```python
from build123d import *

# Parameters (mm, degrees)
BOSS_EXTRUDE2_DEPTH = 3


with BuildPart() as part:
    # Sketch1 → Boss-Extrude2 (new body)
    with BuildSketch(Plane.XY):
        with BuildLine():
            Line((0, 30), (0, 0))
            Line((0, 0), (40, 0))
            add(Edge.make_bspline(
                [(0, 30), (44.385466319, 30.011757551), (40, 0)],
                knots=[0, 0, 0, 1, 1, 1], degree=2))
        make_face()
        with BuildLine():
            Line((11.710831717, 14.823563468), (28.149637062, 14.823563468))
            ThreePointArc((28.149637062, 14.823563468), (33.149637062, 9.823563468), (28.149637062, 4.823563468))
            Line((28.149637062, 4.823563468), (11.710831717, 4.823563468))
            ThreePointArc((11.710831717, 4.823563468), (6.710831717, 9.823563468), (11.710831717, 14.823563468))
        make_face(mode=Mode.SUBTRACT)
    extrude(amount=BOSS_EXTRUDE2_DEPTH)


solid = part.part
```
Geometry: final body of the model. Coordinates: model frame, mm. A direction names the side the tool comes from. Round coordinates to 2 decimals unless told otherwise and drop trailing zeros.
Item 1: Set-up query: faces 1 (the face through (20, 4.824, 1)), 2 (the face through (17, 15, 0)). Return all of +Z, -Z, +X, -X, +Y, -Y with unobstructed straight access to the full face (end or side cutting, diameter ignored); none if empty.
Item 2: Material intervals for L1, parallel to X at y = 4.5, z = 0.55; L2, parallel to Y at x = 17, z = 1; L3, parallel to X at y = 10.5, z = 1, sorted ascending.
Item 3: Mould query, pull axis Y, two halves, no side actions, for faces 3 (the face through (33.15, 9.93, 1.48)), 4 (the face through (6.712, 9.714, 1.479)), 5 (the face through (17, 15, 3)), 6 (the face through (20, 0, 1)). Classes: +Y half, -Y half, draft (parallel to the pull), parting line (faces both ways), or undercut.
Completed:
1. face 1: +Z, -Z
1. face 2: -Z, +X, -X, +Y, -Y
2. L1: x = 0 to 40.39
2. L2: y = 0 to 4.82, 14.82 to 28.58
2. L3: x = 0 to 6.76, 33.1 to 39.87
3. face 3: undercut
3. face 4: undercut
3. face 5: draft
3. face 6: -Y half
